```python
from build123d import *

# Parameters (mm, degrees)
BOSS_EXTRUDE1_DEPTH = 25
CUT_EXTRUDE1_START  = -53
CUT_EXTRUDE1_DEPTH  = 53
SKETCH3_R           = 4
SKETCH3_R_2         = 1
CUT_EXTRUDE2_DEPTH  = 71.295803573
SKETCH4_R           = 4
SKETCH4_R_2         = 1
CUT_EXTRUDE3_DEPTH  = 25
SKETCH5_R           = 1.5
CUT_EXTRUDE4_DEPTH  = 25


# Read off the part's stored shape, not the designer's step: Cut-Extrude1
with BuildPart() as part:
    # Sketch1 → Boss-Extrude1 (new body)
    with BuildSketch(Plane.XY):
        with BuildLine():
            Line((-0.5, 40), (0.5, 40))
            Line((0.5, 40), (0.5, 1.5))
            ThreePointArc((0.5, 1.5), (0.792893219, 0.792893219), (1.5, 0.5))
            Line((1.5, 0.5), (50.5, 0.5))
            ThreePointArc((50.5, 0.5), (51.207106781, 0.792893219), (51.5, 1.5))
            Line((51.5, 1.5), (51.5, 40))
            Line((51.5, 40), (52.5, 40))
            Line((52.5, 40), (52.5, 0.5))
            ThreePointArc((52.5, 0.5), (52.207106781, -0.207106781), (51.5, -0.5))
            Line((51.5, -0.5), (0.5, -0.5))
            ThreePointArc((0.5, -0.5), (-0.207106781, -0.207106781), (-0.5, 0.5))
            Line((-0.5, 0.5), (-0.5, 40))
        make_face()
    extrude(amount=-BOSS_EXTRUDE1_DEPTH)

    # Cut-Extrude1 outline → Cut-Extrude1 (cut)
    with BuildSketch(Plane(origin=(52.5, 0, 0), x_dir=(0, 0, -1), z_dir=(1, 0, 0)).offset(CUT_EXTRUDE1_START)):
        with BuildLine():
            ThreePointArc((0, 27.5), (3.661165235, 36.338834765), (12.5, 40))
            Line((12.5, 40), (0, 40))
            Line((0, 40), (0, 27.5))
        make_face()
        with BuildLine():
            ThreePointArc((12.5, 40), (21.338834765, 36.338834765), (25, 27.5))
            Line((25, 27.5), (25, 40))
            Line((25, 40), (12.5, 40))
        make_face()
    extrude(amount=CUT_EXTRUDE1_DEPTH, mode=Mode.SUBTRACT)

    # Sketch3 → Cut-Extrude2 (cut, through all)
    with BuildSketch(Plane(origin=(0, 0.5, 0), x_dir=(1, 0, 0), z_dir=(0, 1, 0))):
        with Locations(Location((26, 12.5, 0), (0, 0, 270))):
            Circle(SKETCH3_R)
        with Locations(Location((34, 12.5, 0), (0, 0, 270))):
            Circle(SKETCH3_R_2)
        with Locations(Location((26, 20.5, 0), (0, 0, 270))):
            Circle(SKETCH3_R_2)
        with Locations(Location((18, 12.5, 0), (0, 0, 270))):
            Circle(SKETCH3_R_2)
        with Locations(Location((26, 4.5, 0), (0, 0, 270))):
            Circle(SKETCH3_R_2)
    extrude(amount=-CUT_EXTRUDE2_DEPTH, mode=Mode.SUBTRACT)

    # Sketch4 → Cut-Extrude3 (cut)
    with BuildSketch(Plane(origin=(52.5, 0, 0), x_dir=(0, 0, -1), z_dir=(1, 0, 0))):
        with Locations((12.5, 27.5)):
            Circle(SKETCH4_R)
        with Locations((20.5, 27.5)):
            Circle(SKETCH4_R_2)
        with Locations((12.5, 35.5)):
            Circle(SKETCH4_R_2)
        with Locations((12.5, 19.5)):
            Circle(SKETCH4_R_2)
        with Locations((4.5, 27.5)):
            Circle(SKETCH4_R_2)
    extrude(amount=-CUT_EXTRUDE3_DEPTH, mode=Mode.SUBTRACT)

    # Sketch5 → Cut-Extrude4 (cut)
    with BuildSketch(Plane.ZY.offset(0.5)):
        with Locations((-12.5, 27.5)):
            Circle(SKETCH5_R)
    extrude(amount=-CUT_EXTRUDE4_DEPTH, mode=Mode.SUBTRACT)


solid = part.part
```
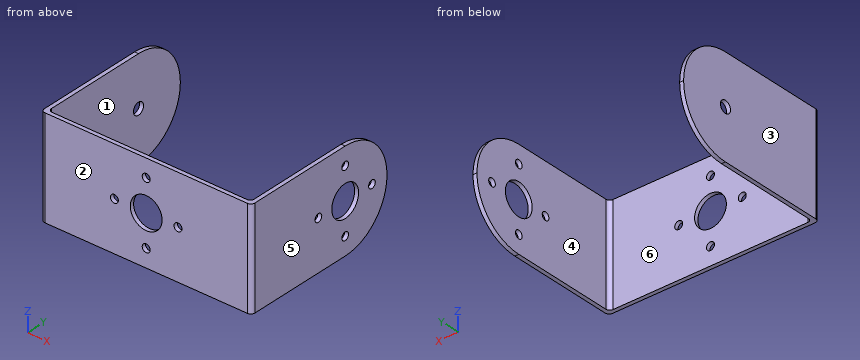
Check sheet for the modelled part. Datum: model origin and axes. Units: mm. Face numbers are marked on the shaded views. A direction names the side the tool comes from. Coordinates: 2 decimals unless noted, no trailing zeros. Write each loop counter-clockwise with the first axis right and the second up, starting at its lowest first coordinate (ties: lowest second). Pieces come first, ordered by that corner, then holes. Notation, with made-up numbers: M 25.25,-27 L 45.25,-27 A12 ccw 45.25,-12 Z; hole C 66,29 d9. An arc over 180 degrees is marked long. Use one line per item in the form item = value.
Item 1: Sectioned sample at C-C, the plane x = 26. Record the cut outline in (y, z).
Answer below:
outline = M -0.5,-25 L 0.5,-25 L 0.5,-21.5 L -0.5,-21.5 Z; M -0.5,-19.5 L 0.5,-19.5 L 0.5,-16.5 L -0.5,-16.5 Z; M -0.5,-8.5 L 0.5,-8.5 L 0.5,-5.5 L -0.5,-5.5 Z; M -0.5,-3.5 L 0.5,-3.5 L 0.5,0 L -0.5,0 Z
Item 2: Sectioned sample at D-D, the plane z = -15. Record the cut outline in (x, y).
Answer below:
outline = M -0.5,0.5 A1 ccw 0.5,-0.5 L 22.88,-0.5 L 22.88,0.5 L 1.5,0.5 A1 cw 0.5,1.5 L 0.5,39.75 L -0.5,39.75 Z; M 29.12,-0.5 L 51.5,-0.5 A1 ccw 52.5,0.5 L 52.5,24.38 L 51.5,24.38 L 51.5,1.5 A1 cw 50.5,0.5 L 29.12,0.5 Z; M 51.5,30.62 L 52.5,30.62 L 52.5,39.75 L 51.5,39.75 Z
Item 3: Release check for a two-part mould opening along X. For the marked faces 1, 2, 3 and 4 record: pulls with the +X half, pulls with the -X half, needs draft (parallel to the pull), parting line crosses it, or undercut.
Answer below:
face_1 = undercut
face_2 = needs draft
face_3 = pulls with the -X half
face_4 = undercut
Item 4: Sectioned sample at B-B, the plane y = 2.5. Record the cut outline in (x, z).
Answer below:
outline = M -0.5,-25 L 0.5,-25 L 0.5,0 L -0.5,0 Z; M 51.5,-25 L 52.5,-25 L 52.5,0 L 51.5,0 Z
Item 5: Gauge pin test, flat ends, axial feed: pin 1 Ø8 at (x, y) = (23.5, 7.5) entering from +Z; pin 2 Ø9 at (x, z) = (26, -12.5) entering from +Y. Record the tip position at first contact, or that the pin passes through.
Answer below:
pin_1 = through
pin_2 = 0.5
Item 6: Sectioned sample at A-A, the plane x = 18. Record the cut outline in (y, z).
Answer below:
outline = M -0.5,-25 L 0.5,-25 L 0.5,-13.5 L -0.5,-13.5 Z; M -0.5,-11.5 L 0.5,-11.5 L 0.5,0 L -0.5,0 Z
Item 7: Set-up check for the marked faces 5 and 6: record each of +Z, -Z, +X, -X, +Y, -Y from which the full face is reachable in a straight line by a thin tool's end or side.
Answer below:
face_5 = +Z, -Z, +X, +Y, -Y
face_6 = +Z, -Z, +Y
Item 8: Material ranges on L1, parallel to X at y = 23.5, z = -23.5; L2, parallel to X at y = 0.1, z = -12.5; L3, parallel to Y at x = 51.95, z = -12.5, recorded low to high. Write a range as from..to.
Answer below:
L1 = -0.5..0.5, 51.5..52.5
L2 = -0.42..17, 19..22, 30..33, 35..52.42
L3 = -0.39..18.5, 20.5..23.5, 31.5..34.5, 36.5..40
